Could you check a few things on this model? Use its own coordinates, in mm. A direction names the side the tool comes from. Give positions to 0.01 mm unless a question says otherwise; leave off trailing zeros. Order: outer loops, then holes, each group sorted by start corner. A loop starts at its lowest first (then second) coordinate and runs counter-clockwise, first axis right, second up. Notation, with made-up numbers: (19, -15.75) -> (59, -15.75) arc R25 ccw to (59, 0.25) -> close; hole circle Ø7 at (-38, 79.25). An arc over 180 degrees is marked (long way). Write each question's results on one line, items separated by ' | '.
```python
from build123d import *

# Parameters (mm, degrees)
F1_DEPTH = 25


with BuildPart() as f1:
    # F0 (on Right) → F1 (new body)
    with BuildSketch(Plane.YZ):
        with BuildLine():
            Line((-29.33908, 7.5), (-32.33908, 7.5))
            Line((-32.33908, 7.5), (-32.33908, -2.5))
            Line((-32.33908, -2.5), (-19.33908, -2.5))
            ThreePointArc((-19.33908, -2.5), (0, -19.5), (19.33908, -2.5))
            Line((19.33908, -2.5), (25.33908, -2.5))
            Line((25.33908, -2.5), (25.33908, 0))
            Line((25.33908, 0), (16.5, 0))
            ThreePointArc((16.5, 0), (0, -16.5), (-16.5, 0))
            Line((-16.5, 0), (-25.33908, 0))
            Line((-25.33908, 0), (-25.33908, 2.5))
            Line((-25.33908, 2.5), (-29.33908, 2.5))
            Line((-29.33908, 2.5), (-29.33908, 7.5))
        make_face()
    extrude(amount=F1_DEPTH)


solid = f1.part
```
Q1. Suppose I cut it at C-C on z = -4.5. Please give me the cut outline in (x, y).
Here are the results:
outline: (0, -18.97) -> (25, -18.97) -> (25, -15.87) -> (0, -15.87) -> close; (0, 15.87) -> (25, 15.87) -> (25, 18.97) -> (0, 18.97) -> close
Q2. For faces 4 (the flat face through (12, 22, -2.5)), 5 (the flat face through (12, -26, -2.5)), 6 (the flat face through (12, 25.339, -1)), 7 (the flat face through (12, -21, 0)), which set-ups out of +Z, -Z, +X, -X, +Y, -Y let a thin tool reach every point of the face, with its end or its side?
Here are the results:
face 4: -Z, +X, -X, +Y | face 5: -Z, +X, -X, -Y | face 6: +Z, -Z, +X, -X, +Y | face 7: +Z, +X, -X, +Y
Q3. Thinking about a two-plate mould opening in Y: for faces 1 (the flat face through (25, -8, -15)), 2 (the flat face through (12, -29.339, 5)), 3 (the cylindrical face through (12.325, 0.363, -16.496)), which applies, +Y half, -Y half, draft (parallel to the pull), parting line (faces both ways), or undercut?
Here are the results:
face 1: draft | face 2: +Y half | face 3: undercut
Q4. I'm going to push flat-ended pins straight in: pin 1 Ø8 at (x, y) = (6, 6) entering from -Z; pin 2 Ø8 at (x, y) = (19.5, 2.5) entering from +Z; pin 3 Ø4.5 at (x, y) = (10, -27) entering from +Z. Where does each tip first touch, or does it pass through?
Here are the results:
pin 1: stops at z = -19.4 | pin 2: stops at z = -15.17 | pin 3: stops at z = 2.5
Q5. I need wall thicknesses on line 1 along Z through (x, y) = (6, -23); line 2 along Y through (x, z) = (8.25, -15); line 3 along Z through (x, y) = (14.75, -26). Which ranges of each line are inside material? Lowest first, please.
Here are the results:
line 1: z = -2.5 to 0 | line 2: y = -12.46 to -6.87, 6.87 to 12.46 | line 3: z = -2.5 to 2.5
Q6. Suppose I cut it at B-B on y = -23. Please give me the cut outline in (x, z).
Here are the results:
outline: (0, -2.5) -> (25, -2.5) -> (25, 0) -> (0, 0) -> close
Q7. Suppose I cut it at D-D on z = 4.25. Please give me the cut outline in (x, y), and give its area (3 significant figures).
Here are the results:
outline: (0, -32.34) -> (25, -32.34) -> (25, -29.34) -> (0, -29.34) -> close | area: 75.0 mm²
Q8. Suppose I cut it at A-A on z = -14.5. Please give me the cut outline in (x, y), and give its area (3 significant figures).
Here are the results:
outline: (0, -13.04) -> (25, -13.04) -> (25, -7.87) -> (0, -7.87) -> close; (0, 7.87) -> (25, 7.87) -> (25, 13.04) -> (0, 13.04) -> close | area: 258 mm²
